Design review of the part built by this model. Coordinates are the model's own, in mm. Face numbers are marked on the shaded views. Coordinates: 2 decimals unless noted, no trailing zeros. Loops run counter-clockwise (first coordinate to the right, second up) from the corner with the lowest first, then second, coordinate; pieces in that order, holes last. Notation, with made-up numbers: M 30.25,-21 L 41.25,-21 A28 cw 41.25,3 Z; hole C 23,-14.5 d8. An arc over 180 degrees is marked long. One line per item, written item: value.
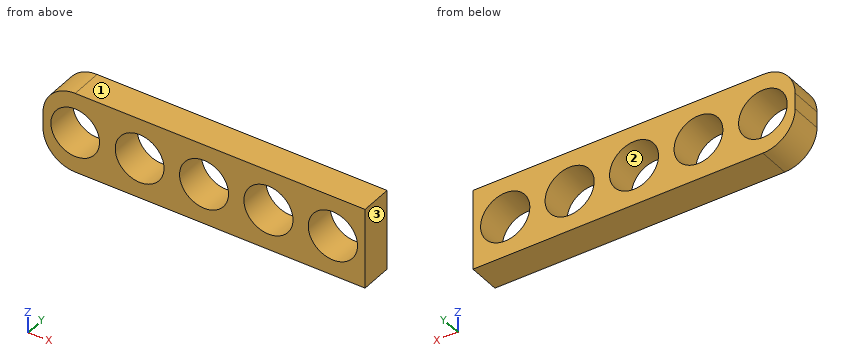
```python
from build123d import *

# Parameters (mm, degrees)
SKETCH1_R           = 7.55
SKETCH1_R_2         = 7.575
SKETCH1_R_3         = 7.6
SKETCH1_R_4         = 7.625
SKETCH1_R_5         = 7.65
BOSS_EXTRUDE1_DEPTH = 10


with BuildPart() as part:
    # Sketch1 → Boss-Extrude1 (new body)
    with BuildSketch(Plane(origin=(0, 0, 0), x_dir=(1, 0, 0), z_dir=(0, 1, 0))):
        with BuildLine():
            Line((-40, 12.5), (50, 12.5))
            Line((50, 12.5), (50, -12.5))
            Line((50, -12.5), (-40, -12.5))
            ThreePointArc((-40, -12.5), (-47.071067812, -9.571067812), (-50, -2.5))
            Line((-50, -2.5), (-50, 2.5))
            ThreePointArc((-50, 2.5), (-47.071067812, 9.571067812), (-40, 12.5))
        make_face()
        with Locations(Location((-40, 0, 0), (0, 0, 270))):
            Circle(SKETCH1_R, mode=Mode.SUBTRACT)
        with Locations(Location((-20, 0, 0), (0, 0, 270))):
            Circle(SKETCH1_R_2, mode=Mode.SUBTRACT)
        with Locations(Location((0, 0, 0), (0, 0, 270))):
            Circle(SKETCH1_R_3, mode=Mode.SUBTRACT)
        with Locations(Location((20, 0, 0), (0, 0, 270))):
            Circle(SKETCH1_R_4, mode=Mode.SUBTRACT)
        with Locations(Location((40, 0, 0), (0, 0, 270))):
            Circle(SKETCH1_R_5, mode=Mode.SUBTRACT)
    extrude(amount=BOSS_EXTRUDE1_DEPTH)


solid = part.part
```
(1) We need section A-A on x = 20. State the section outline as (y, z) points (3 decimals).
Reply:
outline: M 0,-12.5 L 10,-12.5 L 10,-7.625 L 0,-7.625 Z; M 0,7.625 L 10,7.625 L 10,12.5 L 0,12.5 Z
(2) We need section C-C on z = -3.75. State the section outline as (x, y) points.
Reply:
outline: M -49.92,0 L -46.55,0 L -46.55,10 L -49.92,10 Z; M -33.45,0 L -26.58,0 L -26.58,10 L -33.45,10 Z; M -13.42,0 L -6.61,0 L -6.61,10 L -13.42,10 Z; M 6.61,0 L 13.36,0 L 13.36,10 L 6.61,10 Z; M 26.64,0 L 33.33,0 L 33.33,10 L 26.64,10 Z; M 46.67,0 L 50,0 L 50,10 L 46.67,10 Z
(3) To check wall thickness, follow line 1 along X through (y, z) = (3.25, 0.25); line 2 along X through (y, z) = (1, 3.5); line 3 along Z through (x, y) = (40.5, 7.75). State the ranges of each line that lie inside material, in increasing order. Write a range as [from, to].
Reply:
line 1: x = [-50, -47.55], [-32.45, -27.57], [-12.43, -7.6], [7.6, 12.38], [27.62, 32.35], [47.65, 50]
line 2: x = [-49.95, -46.69], [-33.31, -26.72], [-13.28, -6.75], [6.75, 13.23], [26.77, 33.2], [46.8, 50]
line 3: z = [-12.5, -7.63], [7.63, 12.5]
(4) We need section B-B on y = 1.5. State the section outline as (x, z) points (3 decimals), then the cut area to 3 significant figures.
Reply:
outline: M -50,-2.5 A10 ccw -40,-12.5 L 50,-12.5 L 50,12.5 L -40,12.5 A10 ccw -50,2.5 Z; hole C -40,0 d15.1; hole C -20,0 d15.15; hole C 0,0 d15.2; hole C 20,0 d15.25; hole C 40,0 d15.3
area: 1,550 mm2
(5) We need section D-D on x = 0. State the section outline as (y, z) points, then the cut area to 3 significant figures.
Reply:
outline: M 0,-12.5 L 10,-12.5 L 10,-7.6 L 0,-7.6 Z; M 0,7.6 L 10,7.6 L 10,12.5 L 0,12.5 Z
area: 98.0 mm2
(6) Mouldability with a two-part tool opening along X and no side actions: class the marked faces 1, 2 and 3 as released by +X, released by -X, zero draft, split by the parting line, or undercut.
Reply:
face 1: zero draft
face 2: undercut
face 3: released by +X
